Input: dimensioned drawing with shaded views. Units: mm. Origin: part minimum x, y, z. A direction names the side the tool comes from. Round coordinates to 2 decimals unless told otherwise and drop trailing zeros. Order: outer loops, then holes, each group sorted by start corner. A loop starts at its lowest first (then second) coordinate and runs counter-clockwise, first axis right, second up.
Item 1: Cut plane A-A on x = 30. Output: boundary loops of the cut face in (y, z) (1 decimal).
Item 2: Reachability of the marked faces 1 and 2 from +Z, -Z, +X, -X, +Y, -Y: full face, straight path, thin tool, end or side. Return the list, or none.
Item 3: Cut plane B-B on y = 26. Output: boundary loops of the cut face in (x, z).
Item 4: Cut plane D-D on z = 2.5. Give the number of separate pieces and of enclosed holes in the cut face.
Item 5: Mould query, pull axis X, two halves, no side actions, for the marked faces 3 and 4. Classes: released by +X, released by -X, zero draft, split by the parting line, or undercut.
Item 6: First-contact query: pin 1 (0.7 mm diameter, centred on y = 22.5, z = 2.5, fed in from +X); pin 2 (2 mm diameter, centred on y = 42.5, z = 2.5, fed in from -X). Flat tips, straight axial feed; report the tip coordinate or a pass-through.
Item 7: Cut plane C-C on x = 9.5. Output: boundary loops of the cut face in (y, z), then the cut area to 3 significant figures.
Item 8: Line query: L1, parallel to X at y = 13.5, z = 0.7 (1 decimal); L2, parallel to Y at x = 1.4, z = 2.5; L3, parallel to Y at x = 34, z = 1.9 (1 decimal). Output: solid intervals per line, ascending.
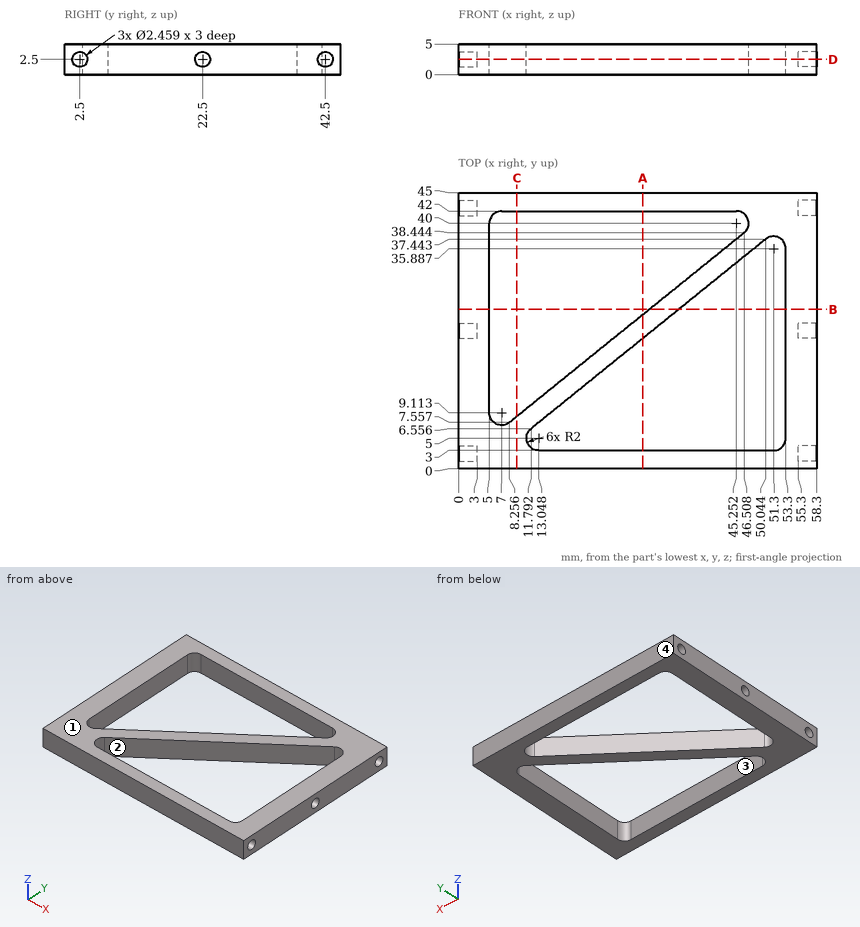
From the geometry:
1. outline: (0, 0) - (3, 0) - (3, 5) - (0, 5) - close; (21.3, 0) - (25.1, 0) - (25.1, 5) - (21.3, 5) - close; (42, 0) - (45, 0) - (45, 5) - (42, 5) - close
2. face 1: +Z, +X, -X, +Y, -Y
2. face 2: +Z, -Z
3. outline: (0, 0) - (5, 0) - (5, 5) - (0, 5) - close; (31.1, 0) - (35.87, 0) - (35.87, 5) - (31.1, 5) - close; (53.3, 0) - (58.3, 0) - (58.3, 5) - (53.3, 5) - close
4. separate pieces: 1
4. enclosed holes: 2
5. face 3: undercut
5. face 4: zero draft
6. pin 1: stops at x = 55.3
6. pin 2: stops at x = 3
7. outline: (0, 0) - (8.56, 0) - (8.56, 5) - (0, 5) - close; (42, 0) - (45, 0) - (45, 5) - (42, 5) - close
7. area: 57.8 mm2
8. L1: x = 0 to 5, 15.6 to 20.4, 53.3 to 58.3
8. L2: y = 0 to 1.27, 3.73 to 21.27, 23.73 to 41.27, 43.73 to 45
8. L3: y = 0 to 3, 24.5 to 28.3, 42 to 45
